from build123d import *

# Parameters (mm, degrees)
SKETCH_1_W          = 120
SKETCH_1_H          = 100
EXTRUDE_1_DEPTH     = 20
SKETCH_1_3_R        = 12.5
CUT_EXTRUDE_2_DEPTH = 10


with BuildPart() as part:
    # 草图1 → 凸台-拉伸1 (new body)
    with BuildSketch(Plane.XY):
        Rectangle(SKETCH_1_W, SKETCH_1_H)
    extrude(amount=EXTRUDE_1_DEPTH)

    # 草图1<3> → 切除-拉伸2 (cut)
    with BuildSketch(Plane.XY):
        Circle(SKETCH_1_3_R)
        with BuildLine():
            Line((-30, -22), (30, -22))
            ThreePointArc((30, -22), (38, -30), (30, -38))
            Line((30, -38), (-30, -38))
            ThreePointArc((-30, -38), (-38, -30), (-30, -22))
        make_face()
    extrude(amount=CUT_EXTRUDE_2_DEPTH, mode=Mode.SUBTRACT)


solid = part.part
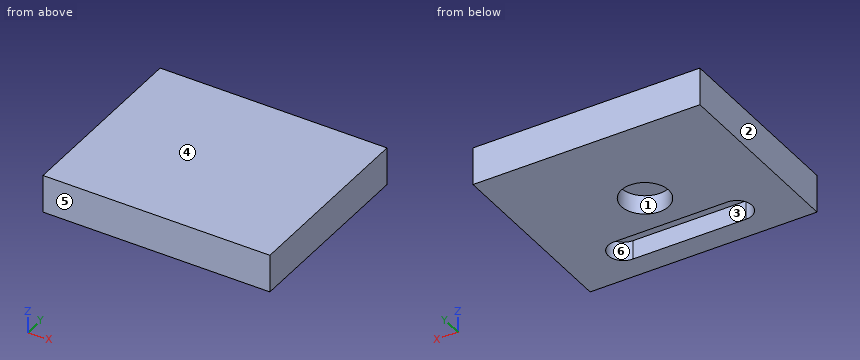
Model file for the job. Use its own axes, mm. Face numbers are marked on the shaded views. A direction names the side the tool comes from. Coordinates: 2 decimals unless noted, no trailing zeros. Order: outer loops, then holes, each group sorted by start corner. A loop starts at its lowest first (then second) coordinate and runs counter-clockwise, first axis right, second up. Notation, with made-up numbers: (-29, 85.25) -> (8, 85.25) arc R32 cw to (8, 117.25) -> close; hole circle Ø5 at (85.5, 69.25). An arc over 180 degrees is marked (long way). Return JSON: item names as keys, results as strings. Group by question number.
Item 1: Pull direction X, two halves, no side cores. Call the marked faces 1, 2, 3 and 4: pulls with the +X half, pulls with the -X half, needs draft (parallel to the pull), parting line crosses it, or undercut.
Item 2: Tool access for the marked faces 5 and 6: list every direction of +Z, -Z, +X, -X, +Y, -Y with a clear straight run to the whole face (end or side of a thin tool).
Item 3: Saw through at B-B on x = -21. Write the cut outline in (y, z).
Item 4: Flat gauge pins, fed straight in: P1, Ø3, axis at x = 32.5, y = -25.5, coming from the -Z side; P2, Ø12, axis at x = -1, y = -11.5, coming from the -Z side. Where does each tip first touch, or does it go through?
Item 5: Saw through at C-C on z = 3.75. Write the cut outline in (x, y).
Item 6: Wall check: line 1 along Y through (x, z) = (0, 8); line 2 along Z through (x, y) = (28, -23.5); line 3 along Y through (x, z) = (35.5, 4). Give the ranges that are in metal, low to high. Write a range as [from, to].
Item 7: Saw through at D-D on x = -8.5. Write the cut outline in (y, z).
Item 8: Saw through at A-A on y = 0. Write the cut outline in (x, z).
Values found:
{
 "1": {"face 1": "undercut", "face 2": "pulls with the -X half", "face 3": "undercut", "face 4": "needs draft"},
 "2": {"face 5": "+Z, -Z, +X, -X, -Y", "face 6": "-Z"},
 "3": {"outline": "(-50, 0) -> (-38, 0) -> (-38, 10) -> (-22, 10) -> (-22, 0) -> (50, 0) -> (50, 20) -> (-50, 20) -> close"},
 "4": {"P1": "stops at z = 10", "P2": "stops at z = 0"},
 "5": {"outline": "(-60, -50) -> (60, -50) -> (60, 50) -> (-60, 50) -> close; hole (-30, -38) -> (30, -38) arc R8 ccw to (30, -22) -> (-30, -22) arc R8 ccw to start; hole circle Ø25 at (0, 0)"},
 "6": {"line 1": "y = [-50, -38], [-22, -12.5], [12.5, 50]", "line 2": "z = [10, 20]", "line 3": "y = [-50, -35.81], [-24.19, 50]"},
 "7": {"outline": "(-50, 0) -> (-38, 0) -> (-38, 10) -> (-22, 10) -> (-22, 0) -> (-9.17, 0) -> (-9.17, 10) -> (9.17, 10) -> (9.17, 0) -> (50, 0) -> (50, 20) -> (-50, 20) -> close"},
 "8": {"outline": "(-60, 0) -> (-12.5, 0) -> (-12.5, 10) -> (12.5, 10) -> (12.5, 0) -> (60, 0) -> (60, 20) -> (-60, 20) -> close"}
}
